from build123d import *

# Parameters (mm, degrees)
SKETCH1_R           = 125
SKETCH1_R_2         = 12.5
BOSS_EXTRUDE1_DEPTH = 40
CUT_EXTRUDE1_REACH  = 183.246
SKETCH2_W           = 12.682043214
SKETCH2_H           = 5.67447182


with BuildPart() as part:
    # Sketch1 → Boss-Extrude1 (new body)
    with BuildSketch(Plane.XY):
        Circle(SKETCH1_R)
        Circle(SKETCH1_R_2, mode=Mode.SUBTRACT)
    extrude(amount=BOSS_EXTRUDE1_DEPTH)

    # Sketch2 → Cut-Extrude1 (cut, up to next)
    with BuildSketch(Plane.XY.offset(40), mode=Mode.PRIVATE) as cut_extrude1_sk1:
        with Locations((0, -11.797375137)):
            Rectangle(SKETCH2_W, SKETCH2_H)
    cut_extrude1_tool1 = extrude(cut_extrude1_sk1.sketch, amount=-CUT_EXTRUDE1_REACH, mode=Mode.PRIVATE) & part.part
    add(cut_extrude1_tool1.solids().sort_by_distance((0, -11.797375, 40))[0], mode=Mode.SUBTRACT)


solid = part.part
Could you check a few things on this model? Use its own coordinates, in mm. Round coordinates to 2 decimals unless told otherwise and drop trailing zeros. Order: outer loops, then holes, each group sorted by start corner. A loop starts at its lowest first (then second) coordinate and runs counter-clockwise, first axis right, second up. Notation, with made-up numbers: M 67.5,-26.75 L 121.5,-26.75 A29 ccw 121.5,11.25 Z; hole C 46,80 d11. An arc over 180 degrees is marked long. One line per item, written item: value.
(1) If we mould it in two halves opening along X, with no side actions, what happens to faces 1 (the flat face through (-2, -26, 0)), 2 (the cylindrical face through (0.46, 12.49, 19.72)), 3 (the cylindrical face through (-124.88, 5.5, 19.72)), 4 (the flat face through (0, -14.635, 20))? For each: released by +X, released by -X, zero draft, split by the parting line, or undercut.
Ans:
face 1: zero draft
face 2: undercut
face 3: split by the parting line
face 4: undercut
(2) I need wall thicknesses on line 1 along X through (y, z) = (-6.5, 31.5); line 2 along Y through (x, z) = (-7, 18.5); line 3 along Y through (x, z) = (8, 34). Which ranges of each line are inside material? Lowest first, please. Write a range as from..to.
Ans:
line 1: x = -124.83..-10.68, 10.68..124.83
line 2: y = -124.8..-10.36, 10.36..124.8
line 3: y = -124.74..-9.6, 9.6..124.74
(3) Imagine slicing it at B-B (y = 0). Write out the boundary of the cut face in (x, z).
Ans:
outline: M -125,0 L -12.5,0 L -12.5,40 L -125,40 Z; M 12.5,0 L 125,0 L 125,40 L 12.5,40 Z
(4) I'm going to push flat-ended pins straight in: P1, Ø5, axis at x = 55.5, z = 30, coming from the -Y side; P2, Ø6, axis at y = 93.5, z = 17, coming from the -X side (3 decimals); P3, Ø1, axis at y = -43, z = 17, coming from the -X side; P4, Ø20, axis at x = 0, y = 0, coming from the -Z side. Where does each tip first touch, or does it pass through?
Ans:
P1: stops at y = -113.21
P2: stops at x = -86.225
P3: stops at x = -117.55
P4: passes through
(5) Imagine slicing it at D-D (y = 54). Write out the boundary of the cut face in (x, z), and give its area (3 significant figures).
Ans:
outline: M -112.73,0 L 112.73,0 L 112.73,40 L -112.73,40 Z
area: 9,020 mm^2
(6) Imagine slicing it at C-C (z = 23). Write out the boundary of the cut face in (x, y), and give its area (3 significant figures).
Ans:
outline: C 0,0 d250; hole M -6.34,-14.63 L 6.34,-14.63 L 6.34,-10.77 A12.5 ccw long -6.34,-10.77 Z
area: 48,600 mm^2
(7) Imagine slicing it at A-A (x = 0). Write out the boundary of the cut face in (y, z).
Ans:
outline: M -125,0 L -14.63,0 L -14.63,40 L -125,40 Z; M 12.5,0 L 125,0 L 125,40 L 12.5,40 Z
